Verification items for the finished model (mm, model axes). A direction names the side the tool comes from. Coordinates: 2 decimals unless noted, no trailing zeros. Order: outer loops, then holes, each group sorted by start corner. A loop starts at its lowest first (then second) coordinate and runs counter-clockwise, first axis right, second up. Notation, with made-up numbers: (29, -40) -> (47, -40) arc R11 ccw to (47, -35) -> close; hole circle Ø3 at (-37.75, 9). An arc over 180 degrees is marked (long way). Answer as CSV lines item,"result".
```python
from build123d import *

# Parameters (mm, degrees)
BOSS_EXTRUDE1_DEPTH = 2
FILLET1_R           = 4


with BuildPart() as part:
    # Sweep3: sweep along a path in Sketch1
    with BuildLine(Plane.XY) as sweep3_path:
        Line((4.5, 18), (4.5, 11.9058809))
        ThreePointArc((4.5, 11.9058809), (5.08127088, 8.723900384), (6.75, 5.95294045))
        ThreePointArc((6.75, 5.95294045), (0, -9), (-6.75, 5.95294045))
        ThreePointArc((-6.75, 5.95294045), (-5.08127088, 8.723900384), (-4.5, 11.9058809))
        Line((-4.5, 11.9058809), (-4.5, 18))
    # Sketch2 → Sweep3 (sweep)
    with BuildSketch(Plane(origin=(-4.5, 18, 0), x_dir=(1, 0, 0), z_dir=(0, 1, 0))):
        with BuildLine():
            Line((0, 3), (0, -3))
            ThreePointArc((0, -3), (-1.757359313, -7.242640687), (-6, -9))
            Line((-6, -9), (-9, -9))
            Line((-9, -9), (-9, -7))
            Line((-9, -7), (-6, -7))
            ThreePointArc((-6, -7), (-3.171572875, -5.828427125), (-2, -3))
            Line((-2, -3), (-2, 3))
            ThreePointArc((-2, 3), (-3.171572875, 5.828427125), (-6, 7))
            Line((-6, 7), (-9, 7))
            Line((-9, 7), (-9, 9))
            Line((-9, 9), (-6, 9))
            ThreePointArc((-6, 9), (-1.757359313, 7.242640687), (0, 3))
        make_face()
    sweep(path=sweep3_path.line)

    # Sketch3 → Boss-Extrude1 (add)
    with BuildSketch(Plane.XY.offset(9)):
        with BuildLine():
            ThreePointArc((-13.5, 11.9058809), (-16.83745824, 6.363961031), (-18, 0))
            Line((-18, 0), (-18, 18))
            Line((-18, 18), (-13.5, 18))
            Line((-13.5, 18), (-13.5, 11.9058809))
        make_face()
        with BuildLine():
            Line((13.5, 18), (13.5, 11.9058809))
            ThreePointArc((13.5, 11.9058809), (16.83745824, 6.363961031), (18, 0))
            Line((18, 0), (18, 18))
            Line((18, 18), (13.5, 18))
        make_face()
    boss_extrude1 = extrude(amount=-BOSS_EXTRUDE1_DEPTH)

    # Mirror2: Boss-Extrude1 across plane
    add(boss_extrude1.mirror(Plane.XY))

    # Fillet1
    fillet1_edges = [part.edges().sort_by_distance(p)[0] for p in [
        (-18, 18, 8),
        (18, 18, 8),
        (-18, 18, -8),
        (18, 18, -8),
    ]]
    fillet(fillet1_edges, radius=FILLET1_R)


solid = part.part
```
Item 1: Section check B-B, the plane x = 0. Record the boundary of the cut face in (y, z), plus the area to 3 significant figures.
Answer list:
outline,"(-18, -9) -> (-15, -9) arc R6 ccw to (-9, -3) -> (-9, 3) arc R6 ccw to (-15, 9) -> (-18, 9) -> (-18, 7) -> (-15, 7) arc R4 cw to (-11, 3) -> (-11, -3) arc R4 cw to (-15, -7) -> (-18, -7) -> close"
area,"55.4 mm2"
Item 2: Tool access check on faces 4 (the cylindrical face through (-6.211, 14.996, -7.196)), 5 (the cylindrical face through (-6.304, 14.996, 7.289)), 6 (the flat face through (13, 8, -7)), 7 (the cylindrical face through (-6.965, 9.398, 0.042)). Record the directions out of +Z, -Z, +X, -X, +Y, -Y that give a thin tool (end or side, any length) a straight path to the whole face; none if there is none.
Answer list:
face 4,"-Z, +Y"
face 5,"+Z, +Y"
face 6,"none"
face 7,"-X, +Y"
Item 3: Section check C-C, the plane z = -1.25. Record the boundary of the cut face in (x, y).
Answer list:
outline,"(-8.25, 7.28) arc R11 ccw (long way) to (8.25, 7.28) arc R7 cw to (6.5, 11.91) -> (6.5, 18) -> (4.5, 18) -> (4.5, 11.91) arc R9 ccw to (6.75, 5.95) arc R9 cw (long way) to (-6.75, 5.95) arc R9 ccw to (-4.5, 11.91) -> (-4.5, 18) -> (-6.5, 18) -> (-6.5, 11.91) arc R7 cw to start"
Item 4: Section check A-A, the plane y = 13. Record the boundary of the cut face in (x, z).
Answer list:
outline,"(-18, -9) -> (-10.5, -9) arc R6 ccw to (-4.5, -3) -> (-4.5, 3) arc R6 ccw to (-10.5, 9) -> (-18, 9) -> (-18, 7) -> (-10.5, 7) arc R4 cw to (-6.5, 3) -> (-6.5, -3) arc R4 cw to (-10.5, -7) -> (-18, -7) -> close; (4.5, -3) arc R6 ccw to (10.5, -9) -> (18, -9) -> (18, -7) -> (10.5, -7) arc R4 cw to (6.5, -3) -> (6.5, 3) arc R4 cw to (10.5, 7) -> (18, 7) -> (18, 9) -> (10.5, 9) arc R6 ccw to (4.5, 3) -> close"
Item 5: Depth check by flat-ended pin: pin 1 Ø1.8 at (y, z) = (14, 0) entering from +X; pin 2 Ø1.8 at (y, z) = (15.5, -1) entering from -X; pin 3 Ø6.5 at (y, z) = (14, 1) entering from -X. Enter the tip coordinate at first touch or a pass-through.
Answer list:
pin 1,"x = 6.5"
pin 2,"x = -6.5"
pin 3,"x = -6.7"
Item 6: Thickness scan on line 1 (Z direction, x = -14.5, y = -8.5); line 2 (X direction, y = 0, z = 1.2); line 3 (Z direction, x = -10.5, y = -7). Record the ranges inside material, lowest first.
Answer list:
line 1,"-9 to -7, 7 to 9"
line 2,"-11 to -9, 9 to 11"
line 3,"-8.51 to -6.21, 6.21 to 8.51"
Item 7: Release check for a two-part mould opening along X. For faces 1 (the flat face through (-6, 18, 1)), 2 (the cylindrical face through (0, -11, 0)), 3 (the flat face through (4.5, 15, 0)) record: +X half, -X half, draft (parallel to the pull), parting line (faces both ways), or undercut.
Answer list:
face 1,"draft"
face 2,"parting line"
face 3,"undercut"
